Design review of the part built by this model. Coordinates are the model's own, in mm. Give positions to 0.01 mm unless a question says otherwise; leave off trailing zeros. Loops run counter-clockwise (first coordinate to the right, second up) from the corner with the lowest first, then second, coordinate; pieces in that order, holes last. Notation, with made-up numbers: (19, 83) -> (24, 83) arc R24 ccw to (24, 102) -> close; hole circle Ø4 at (31.25, 83). An arc over 180 degrees is marked (long way). Use a Markdown table: item, result. Add a question column.
1. Add section D-D (y = 3). State the section outline as (x, z) points, and give its area (3 significant figures).
2. Add section A-A (y = 12.5). State the section outline as (x, z) points.
3. Add section B-B (z = 21.25). State the section outline as (x, y) points.
4. To check wall thickness, follow line 1 (Y direction, x = -12.5, z = 20.2); line 2 (X direction, y = 14, z = 20.75); line 3 (X direction, y = 21.25, z = 21.5). State the ranges of each line that lie inside material, in increasing order.
5. Add section C-C (y = 22.5). State the section outline as (x, z) points, and give its area (3 significant figures).
6. For pin 1 Ø3 at (y, z) = (15, 21) entering from +X, flat-tipped, find the tip position at first contact; note if it passes through.
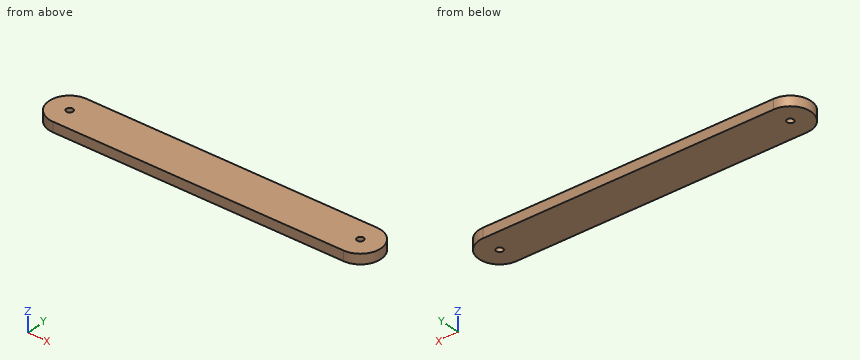
Autodesk Inventor part; units mm, degrees
ref_plane "YZ Plane" through (0, 0, 0) normal (1, 0, 0) x (0, 1, 0)
ref_plane "XZ Plane" through (0, 0, 0) normal (0, 1, 0) x (-1, 0, 0)
ref_plane "XY Plane" through (0, 0, 0) normal (0, 0, 1) x (1, 0, 0)
sketch "Sketch1" plane through (0, 0, 0) normal (0, 0, 1) x (1, 0, 0)
  line L0 (0, 0) -> (-250, 0)
  line L1 (-250, 0) -> (-250, 25)
  line L2 (-250, 25) -> (0, 25)
  line L3 (0, 25) -> (0, 0)
  dimension "d0" = 250
  dimension "d1" = 25
extrude "Extrusion1" add sketch "Sketch1" along normal blind 25
sketch "Sketch3" plane through (0, 0, 25) normal (0, 0, 1) x (1, 0, 0)
  line L0 (0, 25) -> (-250, 25)
  line L1 (-250, 0) -> (0, 0)
  line L2 (-250, 25) -> (-200, 25)
  line L3 (-200, 25) -> (-200, 0)
  line L4 (-200, 0) -> (-250, 0)
  line L5 (-250, 0) -> (-250, 25)
  dimension "d13" = 50
extrude "Extrusion3" cut sketch "Sketch3" against normal blind 25
sketch "Sketch4" plane through (0, 0, 25) normal (0, 0, 1) x (1, 0, 0)
  circle A0 centre (-187.5, 12.5) radius 12.5
  line L0 (-200, 0) -> (0, 0)
  line L1 (-200, 25) -> (-200, 0)
  circle A1 centre (-187.5, 12.5) radius 2
  circle A2 centre (-12.5, 12.5) radius 12.5
  line L2 (0, 0) -> (0, 25)
  circle A3 centre (-12.5, 12.5) radius 2
  line L3 (0, 25) -> (-200, 25)
  point P0 (-12.5, 25)
  point P1 (0, 12.5)
  point P2 (-12.5, 0)
  point P3 (-187.5, 25)
  point P4 (-200, 12.5)
  point P5 (-187.5, 0)
  dimension "d16" = 25
  dimension "d17" = 12.5
  dimension "d18" = 12.5
  dimension "d19" = 4
  dimension "d20" = 25
  dimension "d21" = 12.5
  dimension "d22" = 12.5
  dimension "d23" = 4
extrude "Extrusion4" cut sketch "Sketch4" against normal blind 25 contours A0 L1 L3 | L0 L1 A0 | L3 L2 A2 | A2 L2 L0 | A1 | A3
sketch "Sketch5" plane through (-187.5, 25, 0) normal (0, 1, 0) x (1, 0, 0)
  line L0 (-12.5, 0) -> (-12.5, -25)
  line L1 (187.5, 0) -> (-12.5, 0)
  line L2 (-12.5, 0) -> (-12.5, -19)
  line L3 (-12.5, -19) -> (187.5, -19)
  line L4 (187.5, -19) -> (187.5, 0)
  dimension "d26" = 19
extrude "Extrusion5" cut sketch "Sketch5" against normal blind 100
properties part number "Horizontal"
Taken from the geometry:
| question | item | result |
|---|---|---|
| 1 | outline | (-195.62, 19) -> (-4.38, 19) -> (-4.38, 25) -> (-195.62, 25) -> close |
| 1 | area | 1,150 mm^2 |
| 2 | outline | (-200, 19) -> (-189.5, 19) -> (-189.5, 25) -> (-200, 25) -> close; (-185.5, 19) -> (-14.5, 19) -> (-14.5, 25) -> (-185.5, 25) -> close; (-10.5, 19) -> (0, 19) -> (0, 25) -> (-10.5, 25) -> close |
| 3 | outline | (-187.5, 0) -> (-12.5, 0) arc R12.5 ccw to (-12.5, 25) -> (-187.5, 25) arc R12.5 ccw to start; hole circle Ø4 at (-187.5, 12.5); hole circle Ø4 at (-12.5, 12.5) |
| 4 | line 1 | y = 0 to 10.5, 14.5 to 25 |
| 4 | line 2 | x = -199.91 to -188.82, -186.18 to -13.82, -11.18 to -0.09 |
| 4 | line 3 | x = -196.43 to -3.57 |
| 5 | outline | (-195, 19) -> (-5, 19) -> (-5, 25) -> (-195, 25) -> close |
| 5 | area | 1,140 mm^2 |
| 6 | pin 1 | stops at x = -0.04 |
